```python
from build123d import *

# Parameters (mm, degrees)
CUT_EXTRUDE1_DEPTH      = 66.493994813
CUT_EXTRUDE1_DEPTH_BACK = 66.493994813
SKETCH2_R               = 7.9375


with BuildPart() as part:
    # Sketch1 → Revolve1 (revolve)
    with BuildSketch(Plane.XY, mode=Mode.PRIVATE) as revolve1_sk:
        Polygon((19.05, -11.8872), (19.05, -13.2842), (20.447, -11.8872), align=None)
        with BuildLine():
            ThreePointArc((5.771901147, -14.059921768), (7.048009176, -9.297421768), (10.534401147, -5.811029797))
            Line((10.534401147, -5.811029797), (20.5994, 0))
            Line((20.5994, 0), (23.7744, 0))
            Line((23.7744, 0), (23.7744, -6.9342))
            Line((23.7744, -6.9342), (25.2095, -6.9342))
            Line((25.2095, -6.9342), (25.2095, -10.1092))
            Line((25.2095, -10.1092), (22.2123, -10.1092))
            Line((22.2123, -10.1092), (22.2123, -11.8872))
            Line((22.2123, -11.8872), (19.05, -11.8872))
            Line((19.05, -11.8872), (19.05, -54.9402))
            Line((19.05, -54.9402), (15.875, -54.9402))
            Line((15.875, -54.9402), (5.771901147, -17.234921768))
            Line((5.771901147, -17.234921768), (5.771901147, -14.059921768))
        make_face()
    revolve(revolve1_sk.sketch.rotate(Axis((0, 0, 0), (0, 1, 0)), 90), axis=Axis((0, 0, 0), (0, 1, 0)))

    # Sketch2 → Cut-Extrude1 (cut, two sides: drawn at the far end of the back side and taken through both)
    with BuildSketch(Plane(origin=(0, 0, 0), x_dir=(1, 0, 0), z_dir=(0, 1, 0)).offset(-CUT_EXTRUDE1_DEPTH_BACK)):
        with Locations(Location((0, 0, 0), (0, 0, 90))):
            Circle(SKETCH2_R)
    extrude(amount=CUT_EXTRUDE1_DEPTH + CUT_EXTRUDE1_DEPTH_BACK, mode=Mode.SUBTRACT)


solid = part.part
```
Geometry: final body of the model. Coordinates: model frame, mm. A direction names the side the tool comes from. Give positions to 0.01 mm unless a question says otherwise; leave off trailing zeros. Order: outer loops, then holes, each group sorted by start corner. A loop starts at its lowest first (then second) coordinate and runs counter-clockwise, first axis right, second up. Notation, with made-up numbers: (45, 66) -> (76, 66) arc R25 ccw to (76, 105) -> close; hole circle Ø5 at (82.25, 47). An arc over 180 degrees is marked (long way). Write each question's results on one line, items separated by ' | '. Start each with the question number.
1) Set-up query: faces 4 (the flat face through (22.3, -10.109, -1.7)), 5 (the cylindrical face through (7.75, -16.79, 1.72)), 6 (the cylindrical face through (-7.141, -3.516, -22.677)). Return all of +Z, -Z, +X, -X, +Y, -Y with unobstructed straight access to the full face (end or side cutting, diameter ignored); none if empty.
2) Draft query along X for faces 1 (the conical face through (-3.353, -5.448, -10.648)), 2 (the flat face through (6, -11.887, -20)), 3 (the cylindrical face through (18.597, -34.404, 4.13)). Return one class per face: pulls with the +X half, pulls with the -X half, needs draft (parallel to the pull), parting line crosses it, or undercut.
3) Line query: line 1 (X direction, y = -20.5, z = 0); line 2 (Y direction, x = -8.5, z = 22); line 3 (Z direction, x = 5, y = -32.5). Output: solid intervals per line, ascending. Write a range as from..to.
4) First-contact query: pin 1 (1 mm diameter, centred on x = 13.5, y = -39, fed in from -Z); pin 2 (12 mm diameter, centred on x = 5.5, z = 3, fed in from +Y); pin 3 (8 mm diameter, centred on y = -5.5, z = -15, fed in from -X). Flat tips, straight axial feed; report the tip coordinate or a pass-through.
5) Section D-D (y = -4.5). Return loops of the section in (x, z), then the cut area to 3 significant figures.
Calculated:
1) face 4: -Y | face 5: +Y, -Y | face 6: +Y
2) face 1: undercut | face 2: needs draft | face 3: parting line crosses it
3) line 1: -19.05..-7.94, 7.94..19.05 | line 2: -10.11..0 | line 3: -18.38..-8.5, 8.5..18.38
4) pin 1: z = -13.92 | pin 2: y = -4.81 | pin 3: x = -22.55
5) outline: circle Ø47.55 at (0, 0); hole circle Ø25.61 at (0, 0) | area: 1,260 mm2
